```python
from build123d import *

# Parameters (mm, degrees)
F0_W       = 20
F0_H       = 25
F1_DEPTH   = 5
F2_W       = 20
F2_H       = 5
F3_DEPTH   = 20
F6_D       = 3.2
F6_ON_F5_D = 3.2
F7_W       = 20
F7_H       = 5
F8_DEPTH   = 25
F9_R       = 1.6
F9_R_2     = 12.5
F10_DEPTH  = 5


with BuildPart() as f1:
    # F0 (on Front) → F1 (new body)
    with BuildSketch(Plane.XZ):
        with Locations((10, 12.5)):
            Rectangle(F0_W, F0_H)
    extrude(amount=F1_DEPTH)

    # F2 (on face) → F3 (join)
    with BuildSketch(Plane(origin=(0, 0, 0), x_dir=(-1, 0, 0), z_dir=(0, 1, 0))):
        with Locations((-10, 22.5)):
            Rectangle(F2_W, F2_H)
    extrude(amount=F3_DEPTH)

    # F6 (through all)
    with Locations(Plane(origin=(0, 0, 0), x_dir=(-1, 0, 0), z_dir=(0, 1, 0))):
        with Locations((-10, 10)):
            Hole(F6_D / 2)

    # F6 on F5 (through all)
    with Locations(Plane(origin=(0, 0, 20), x_dir=(1, 0, 0), z_dir=(0, 0, -1))):
        with Locations((10, -10)):
            Hole(F6_ON_F5_D / 2)

    # F7 (on face) → F8 (join)
    with BuildSketch(Plane.XY.offset(25)):
        with Locations((10, 22.5)):
            Rectangle(F7_W, F7_H)
    extrude(amount=-F8_DEPTH)

    # F9 (on face) → F10 (join)
    with BuildSketch(Plane(origin=(0, 0, 0), x_dir=(0, -1, 0), z_dir=(-1, 0, 0))):
        Polygon((7.65, 27), (7.65, 69.3), (-34.65, 69.3), (-34.65, 27), (-25, 0), (-20, 0), (-20, 20), (0, 20), (0, 0), (5, 0), align=None)
        with Locations((-29, 32.65)):
            Circle(F9_R, mode=Mode.SUBTRACT)
        with Locations((2, 32.65)):
            Circle(F9_R, mode=Mode.SUBTRACT)
        with Locations((-29, 63.65)):
            Circle(F9_R, mode=Mode.SUBTRACT)
        with Locations((-13.5, 48.15)):
            Circle(F9_R_2, mode=Mode.SUBTRACT)
        with Locations((2, 63.65)):
            Circle(F9_R, mode=Mode.SUBTRACT)
    extrude(amount=F10_DEPTH)


solid = f1.part
```
Work out the finished part from the listing and answer in its coordinate system (mm). A direction names the side the tool comes from. Round coordinates to 2 decimals unless told otherwise and drop trailing zeros. Write each loop counter-clockwise with the first axis right and the second up, starting at its lowest first coordinate (ties: lowest second). Pieces come first, ordered by that corner, then holes. Notation, with made-up numbers: (63, -35) - (74, -35) arc R11 cw to (74, -17) - close; hole circle Ø11 at (55.25, 85.25). An arc over 180 degrees is marked (long way). Return JSON: item names as keys, results as strings. Group by question number.
Q1. The part is cut by section C-C on y = 10. Write down the section's boundary in (x, z), then the cut area to 4 significant figures.
Q2. The part is cut by section B-B on x = -1.75. Write down the section's boundary in (y, z), then the cut area to 3 significant figures.
Q3. For faces 5 (the flat face through (10, -5, 13)), 6 (the flat face through (8, 10, 20)), 7 (the flat face through (10, 25, 13)), 8 (the cylindrical face through (11.27, 10.97, 22.54)), determine the directions among +Z, -Z, +X, -X, +Y, -Y from which every point of the face is accessible in a straight line to the end or side of a thin tool.
Q4. The mould has two halves that part along Z. Classify faces 1 (the flat face through (20, 6, 21)), 2 (the cylindrical face through (-2.46, 29.35, 31.09)), 3 (the cylindrical face through (-2.46, 29.35, 62.09)), 4 (the flat face through (12, 10, 25)): released by +Z, released by -Z, zero draft, split by the parting line, or undercut.
Q5. The part is cut by section A-A on y = -2. Write down the section's boundary in (x, z), then the cut area to 3 significant figures.
Q6. Find the intervals of material crossed by L1, parallel to Z at x = -2.2, y = -2; L2, parallel to Y at x = 5, z = 5; L3, parallel to X at y = 10, z = 21.5, in increasing order.
Q7. Each of these flat-tipped pins is pushed along its axis until it touches: pin 1 Ø1.9 at (x, z) = (10, 10) entering from +Y; pin 2 Ø3.5 at (y, z) = (29, 63.65) entering from +X; pin 3 Ø10 at (x, y) = (8.5, 12.5) entering from -Z. Where does it stop, or does it pass through?
Q8. The part is cut by section D-D on x = 10. Write down the section's boundary in (y, z).
Solved:
{
 "1": {"outline": "(-5, 20) - (8.4, 20) - (8.4, 25) - (0, 25) - (0, 36.15) - (-5, 36.15) - close; (-5, 60.15) - (0, 60.15) - (0, 69.3) - (-5, 69.3) - close; (11.6, 20) - (20, 20) - (20, 25) - (11.6, 25) - close", "area": "210.5 mm²"},
 "2": {"outline": "(-7.65, 27) - (-5, 0) - (0, 0) - (0, 20) - (20, 20) - (20, 0) - (25, 0) - (34.65, 27) - (34.65, 69.3) - (-7.65, 69.3) - close; hole circle Ø3.2 at (-2, 32.65); hole circle Ø3.2 at (-2, 63.65); hole circle Ø25 at (13.5, 48.15); hole circle Ø3.2 at (29, 32.65); hole circle Ø3.2 at (29, 63.65)", "area": "1,840 mm²"},
 "3": {"face 5": "+Z, -Z, +X, -Y", "face 6": "-Z, +X, -X", "face 7": "+Z, -Z, +X, +Y", "face 8": "+Z, -Z"},
 "4": {"face 1": "zero draft", "face 2": "undercut", "face 3": "undercut", "face 4": "released by +Z"},
 "5": {"outline": "(-5, 0) - (20, 0) - (20, 25) - (0, 25) - (0, 31.05) - (-5, 31.05) - close; (-5, 34.25) - (0, 34.25) - (0, 62.05) - (-5, 62.05) - close; (-5, 65.25) - (0, 65.25) - (0, 69.3) - (-5, 69.3) - close; hole circle Ø3.2 at (10, 10)", "area": "806 mm²"},
 "6": {"L1": "0 to 31.05, 34.25 to 62.05, 65.25 to 69.3", "L2": "-5 to 0, 20 to 25", "L3": "-5 to 8.4, 11.6 to 20"},
 "7": {"pin 1": "y = 25", "pin 2": "x = 0", "pin 3": "z = 20"},
 "8": {"outline": "(-5, 0) - (0, 0) - (0, 8.4) - (-5, 8.4) - close; (-5, 11.6) - (0, 11.6) - (0, 20) - (8.4, 20) - (8.4, 25) - (-5, 25) - close; (11.6, 20) - (20, 20) - (20, 0) - (25, 0) - (25, 25) - (11.6, 25) - close"}
}
